from build123d import *

# Parameters (mm, degrees)
F0_W     = 25.4
F0_H     = 13.97
F1_DEPTH = 63.5


with BuildPart() as f1:
    # F0 (on Front) → F1 (new body, symmetric)
    with BuildSketch(Plane.XZ):
        with BuildLine():
            add(Edge.make_bspline(
                [(-41.275, 9.525), (-38.7320481241, 45.0227931142), (26.9261933863, 64.3182843924), (57.15, 66.675)],
                knots=[0, 0, 0, 0, 113.8138968887, 113.8138968887, 113.8138968887, 113.8138968887], degree=3))
            Line((-41.275, 9.525), (27.305, 9.525))
            Line((27.305, 9.525), (27.305, 36.5125))
            ThreePointArc((27.305, 36.5125), (36.0463981155, 57.6161018845), (57.15, 66.3575))
            Line((57.15, 66.3575), (57.15, 66.675))
        make_face()
        Polygon((27.305, 9.525), (-41.275, 9.525), (-41.275, -9.525), (41.275, -9.525), (41.275, 9.525), align=None)
        with BuildLine():
            Line((27.305, 36.5125), (27.305, 9.525))
            Line((27.305, 9.525), (41.275, 9.525))
            Line((41.275, 9.525), (41.275, 36.5125))
            ThreePointArc((41.275, 36.5125), (45.9246798487, 47.7378201513), (57.15, 52.3875))
            Line((57.15, 52.3875), (57.15, 66.3575))
            ThreePointArc((57.15, 66.3575), (36.0463981155, 57.6161018845), (27.305, 36.5125))
        make_face()
        Polygon((107.95, 66.675), (57.15, 66.675), (57.15, 66.3575), (82.55, 66.3575), (82.55, 52.3875), (57.15, 52.3875), (57.15, 38.1), (107.95, 38.1), align=None)
        with Locations((69.85, 59.3725)):
            Rectangle(F0_W, F0_H)
    extrude(amount=F1_DEPTH, both=True)


solid = f1.part
The listing builds one solid part. Answer for the finished solid, in the listing's coordinates (mm). A direction names the side the tool comes from. Coordinates: 2 decimals unless noted, no trailing zeros. Write each loop counter-clockwise with the first axis right and the second up, starting at its lowest first coordinate (ties: lowest second). Pieces come first, ordered by that corner, then holes. Notation, with made-up numbers: (7.25, -36.75) - (34.25, -36.75) arc R25 cw to (34.25, -18.75) - close; hole circle Ø11 at (-18.5, 28). An arc over 180 degrees is marked (long way). Return JSON: item names as keys, results as strings.
1. The part is cut by section A-A on z = -4. Determine the outline of the cut face in (x, y) (3 decimals).
Final values:
{"outline": "(-41.275, -63.5) - (41.275, -63.5) - (41.275, 63.5) - (-41.275, 63.5) - close"}
2. The part is cut by section B-B on x = 66.5. Determine the outline of the cut face in (y, z) (3 decimals).
Final values:
{"outline": "(-63.5, 38.1) - (63.5, 38.1) - (63.5, 66.675) - (-63.5, 66.675) - close"}
3. Which of the six approach directions +Z, -Z, +X, -X, +Y, -Y give full straight-line access (tool end or side, diameter ignored) to faces 1 (the face through (45.8, -0.89, 47.61)), 2 (the face through (83, -1, 66.675)), 3 (the face through (82, -1, 38.1))?
Final values:
{"face 1": "-Z, +Y, -Y", "face 2": "+Z, +X, -X, +Y, -Y", "face 3": "-Z, +X, +Y, -Y"}
4. Consider line 1 along X through (y, z) = (-11, -3) (3 decimals); line 2 along Z through (x, y) = (93.5, -24) (3 decimals); line 3 along X through (y, z) = (48, 42.5). Determine where each line is inside the solid, lowest interval first.
Final values:
{"line 1": "-41.275 to 41.275", "line 2": "38.1 to 66.675", "line 3": "-17.12 to 42.45, 57.15 to 107.95"}
5. Each of these flat-tipped pins is pushed along its axis until it touches: pin 1 Ø6 at (x, y) = (28.5, -7.5) entering from +Z; pin 2 Ø11.5 at (y, z) = (-14, 44.5) entering from -X; pin 3 Ø5 at (x, z) = (82, 37) entering from +Y; pin 4 Ø4 at (x, y) = (-10, 12) entering from +Z. Where does it stop, or does it pass through?
Final values:
{"pin 1": "z = 62.28", "pin 2": "x = -22.48", "pin 3": "y = 63.5", "pin 4": "z = 47.79"}
6. For a pull along X with two mould halves and no side action, classify faces 4 (the face through (-41.275, -1, 0)), 5 (the face through (107.95, -1, 52)), 6 (the face through (57.15, -1, 45)) as +X half, -X half, draft (parallel to the pull), parting line (faces both ways), or undercut.
Final values:
{"face 4": "-X half", "face 5": "+X half", "face 6": "undercut"}
